Geometry check sheet. Reference: the model listing, model coordinates, mm. A direction names the side the tool comes from. Coordinates: 2 decimals unless noted, no trailing zeros. Loops run counter-clockwise (first coordinate to the right, second up) from the corner with the lowest first, then second, coordinate; pieces in that order, holes last. Notation, with made-up numbers: (76, -33.75) -> (92, -33.75) arc R30 ccw to (92, 0.25) -> close; hole circle Ø6 at (-33, 61.25). An arc over 180 degrees is marked (long way). Answer as a JSON object with one key per item and string values.
from build123d import *

# Parameters (mm, degrees)
F2_DEPTH  = 45
F4_DEPTH  = 10
F6_T      = -2
F5_W      = 71.5
F5_H      = 24.5
F7_DEPTH  = 2
F9_DEPTH  = 2.7
F11_DEPTH = 2


with BuildPart() as f2:
    # F1 (on Right) → F2 (new body, symmetric)
    with BuildSketch(Plane.YZ):
        Polygon((51.6187950266, -51.6187950266), (0, 0), (0, -97.2855082581), (51.6187950266, -97.2855082581), align=None)
    extrude(amount=F2_DEPTH, both=True)

    # F3 (on face) → F4 (join)
    with BuildSketch(Plane(origin=(-45, 0, 0), x_dir=(0, -1, 0), z_dir=(-1, 0, 0))):
        Polygon((-51.6187950266, -51.6187950266), (-51.6187950266, -97.2855082581), (0, -97.2855082581), (0, 0), align=None)
    extrude(amount=F4_DEPTH)

    # F6
    f6_openings = [f2.faces().sort_by_distance(p)[0] for p in [
        (-5, 0, -48.642754),
    ]]
    offset(amount=F6_T, openings=f6_openings)

    # F5 (on face) → F7 (cut, through all)
    with BuildSketch(Plane(origin=(0, 0, 0), x_dir=(-1, 0, 0), z_dir=(0, 0.7071067812, 0.7071067812))):
        with Locations((0, -51.5)):
            Rectangle(F5_W, F5_H)
    extrude(amount=-F7_DEPTH, mode=Mode.SUBTRACT)

    # F8 (on face) → F9 (join)
    with BuildSketch(Plane(origin=(0, -1.4142135624, -1.4142135624), x_dir=(1, 0, 0), z_dir=(0, -0.7071067812, -0.7071067812))):
        Polygon((-32.75, -63.8013684387), (-34.75, -63.8013684387), (-34.75, -65.4756842194), (-34.75, -68.8243157807), (-37.65, -70.4986315613), (-40.55, -68.8243157807), (-40.55, -65.4756842194), (-40.55, -63.8013684387), (-42.55, -63.8013684387), (-42.55, -72.1715728753), (-32.75, -72.1715728753), align=None)
        Polygon((-40.55, -32.5013684387), (-42.55, -32.5013684387), (-42.55, -39.25), (-42.55, -41.25), (-35.75, -41.25), (-35.75, -39.25), (-32.75, -39.25), (-32.75, -32.5013684387), (-34.75, -32.5013684387), (-34.75, -37.5243157807), (-37.65, -39.1986315613), (-40.55, -37.5243157807), align=None)
        Polygon((32.75, -32.5013684387), (32.75, -39.25), (35.75, -39.25), (35.75, -41.25), (42.55, -41.25), (42.55, -39.25), (42.55, -32.5013684387), (40.55, -32.5013684387), (40.55, -37.5243157807), (37.65, -39.1986315613), (34.75, -37.5243157807), (34.75, -32.5013684387), align=None)
        Polygon((34.75, -65.4756842194), (34.75, -63.8013684387), (32.75, -63.8013684387), (32.75, -72.1715728753), (42.55, -72.1715728753), (42.55, -63.8013684387), (40.55, -63.8013684387), (40.55, -65.4756842194), (40.55, -68.8243157807), (37.65, -70.4986315613), (34.75, -68.8243157807), align=None)
    extrude(amount=F9_DEPTH)

    # F10 (on face) → F11 (join)
    with BuildSketch(Plane(origin=(0, -3.3234018716, -3.3234018716), x_dir=(1, 0, 0), z_dir=(0, -0.7071067812, -0.7071067812))):
        Polygon((-42.55, -32.5013684387), (-42.55, -41.25), (-35.75, -41.25), (-35.75, -39.25), (-32.75, -39.25), (-32.75, -32.5013684387), align=None)
        Polygon((32.75, -39.25), (35.75, -39.25), (35.75, -41.25), (42.55, -41.25), (42.55, -32.5013684387), (40.55, -32.5013684387), (40.55, -37.5243157807), (37.65, -39.1986315613), (34.75, -37.5243157807), (34.75, -32.5013684387), (32.75, -32.5013684387), align=None)
        Polygon((40.55, -32.5013684387), (34.75, -32.5013684387), (34.75, -37.5243157807), (37.65, -39.1986315613), (40.55, -37.5243157807), align=None)
        Polygon((37.65, -70.4986315613), (34.75, -68.8243157807), (34.75, -63.8013684387), (32.75, -63.8013684387), (32.75, -72.1715728753), (42.55, -72.1715728753), (42.55, -63.8013684387), (40.55, -63.8013684387), (40.55, -68.8243157807), align=None)
        Polygon((34.75, -63.8013684387), (34.75, -68.8243157807), (37.65, -70.4986315613), (40.55, -68.8243157807), (40.55, -63.8013684387), align=None)
        Polygon((-42.55, -72.1715728753), (-32.75, -72.1715728753), (-32.75, -63.8013684387), (-34.75, -63.8013684387), (-34.75, -68.8243157807), (-37.65, -70.4986315613), (-40.55, -68.8243157807), (-40.55, -63.8013684387), (-42.55, -63.8013684387), align=None)
        Polygon((-34.75, -68.8243157807), (-34.75, -63.8013684387), (-40.55, -63.8013684387), (-40.55, -68.8243157807), (-37.65, -70.4986315613), align=None)
    extrude(amount=F11_DEPTH)


solid = f2.part
1. Section check B-B, the plane z = -63. Record the boundary of the cut face in (x, y), then the cut area to 3 significant figures.
Evaluation:
{"outline": "(-55, 0) -> (-53, 0) -> (-53, 49.62) -> (43, 49.62) -> (43, 0) -> (45, 0) -> (45, 51.62) -> (-55, 51.62) -> close", "area": "398 mm^2"}
2. Tool access check on faces 1 (the face through (-32.75, 22, -28)), 2 (the face through (-0.17, 26.8, -28.71)), 3 (the face through (34.75, 45, -49)). Record the directions out of +Z, -Z, +X, -X, +Y, -Y that give a thin tool (end or side, any length) a straight path to the whole face; none if there is none.
Evaluation:
{"face 1": "-Y", "face 2": "+Y", "face 3": "none"}
3. Mould release check, pull along Z, two halves, no side actions. Record for faces 4 (the face through (-55, 20, -59)), 5 (the face through (37.581, 21.294, -30.769)): released by +Z, released by -Z, zero draft, split by the parting line, or undercut.
Evaluation:
{"face 4": "zero draft", "face 5": "undercut"}
4. Section check D-D, the plane y = 8. Record the boundary of the cut face in (x, z).
Evaluation:
{"outline": "(-55, -97.29) -> (45, -97.29) -> (45, -8) -> (-55, -8) -> close; hole (-53, -95.29) -> (43, -95.29) -> (43, -10.83) -> (-53, -10.83) -> close"}
5. Thickness scan on probe 1 along X at (y, z) = (33, -91); probe 2 along Y at (x, z) = (6, -73.5); probe 3 along Z at (x, y) = (8, 19). Record the ranges inside material, lowest first. Write a range as from..to.
Evaluation:
{"probe 1": "x = -55..-53, 43..45", "probe 2": "y = 49.62..51.62", "probe 3": "z = -97.29..-95.29, -21.83..-19"}
6. Section check C-C, the plane y = 30.5. Record the boundary of the cut face in (x, z).
Evaluation:
{"outline": "(-55, -97.29) -> (45, -97.29) -> (45, -30.5) -> (35.75, -30.5) -> (35.75, -33.33) -> (43, -33.33) -> (43, -95.29) -> (-53, -95.29) -> (-53, -33.33) -> (-35.75, -33.33) -> (-35.75, -30.5) -> (-55, -30.5) -> close"}
7. Depth check by flat-ended pin: P1, Ø3, axis at x = -39.5, z = -19.5, coming from the -Y side; P2, Ø10, axis at x = 8, z = -34.5, coming from the +Y side; P3, Ø1.5, axis at x = 27, y = 22, coming from the +Z side. Enter the tip coordinate at first touch or a pass-through.
Evaluation:
{"P1": "stops at y = 15.17", "P2": "passes through", "P3": "stops at z = -21.25"}
8. Section check A-A, the plane x = 4.5. Record the boundary of the cut face in (y, z).
Evaluation:
{"outline": "(0, -97.29) -> (51.62, -97.29) -> (51.62, -51.62) -> (45.08, -45.08) -> (43.66, -46.49) -> (49.62, -52.45) -> (49.62, -95.29) -> (0, -95.29) -> close; (0, -2.83) -> (26.34, -29.17) -> (27.75, -27.75) -> (0, 0) -> close"}
